```python
from build123d import *

# Parameters (mm, degrees)
ESQUISSE1_W                  = 38
ESQUISSE1_H                  = 36
BOSS_EXTRU_1_DEPTH           = 3
BOSS_EXTRU_2_DEPTH           = 10
ENL_V_MAT_EXTRU_1_DEPTH      = 54.935146241
ENL_V_MAT_EXTRU_1_DEPTH_BACK = 54.935146241
ESQUISSE4_R                  = 0.75
ENL_V_MAT_EXTRU_2_DEPTH      = 19.8
ENL_V_MAT_EXTRU_3_DEPTH      = 54.935146241
ENL_V_MAT_EXTRU_3_DEPTH_BACK = 54.935146241
ESQUISSE5_R                  = 0.75
BOSS_EXTRU_3_START           = -2.6
BOSS_EXTRU_3_DEPTH           = 30.8
BOSS_EXTRU_4_START           = -19.8
BOSS_EXTRU_4_DEPTH           = 19.8


with BuildPart() as part:
    # Esquisse1 → Boss.-Extru.1 (new body)
    with BuildSketch(Plane.XY):
        with Locations((19, 18)):
            Rectangle(ESQUISSE1_W, ESQUISSE1_H)
    extrude(amount=BOSS_EXTRU_1_DEPTH)

    # Esquisse2 → Boss.-Extru.2 (add)
    with BuildSketch(Plane.XY.offset(3)):
        Polygon((38, 33.1), (3, 33.1), (3, 2.9), (38, 2.9), (38, 0), (0, 0), (0, 36), (38, 36), align=None)
    extrude(amount=BOSS_EXTRU_2_DEPTH)

    # Esquisse3 → Enlèv. mat.-Extru.1 (cut, two sides: drawn at the far end of the back side and taken through both)
    with BuildSketch(Plane(origin=(0, 0, 0), x_dir=(-1, 0, 0), z_dir=(0, 0, -1)).offset(-ENL_V_MAT_EXTRU_1_DEPTH_BACK)):
        Polygon((0, 2.6), (0, 0), (-18.2, 0), (-18.2, 5.809151049), align=None)
        Polygon((-18.2, 36), (-18.2, 30.190848951), (0, 33.4), (0, 36), align=None)
    extrude(amount=ENL_V_MAT_EXTRU_1_DEPTH + ENL_V_MAT_EXTRU_1_DEPTH_BACK, mode=Mode.SUBTRACT)

    # Esquisse4 → Enlèv. mat.-Extru.2 (cut)
    with BuildSketch(Plane(origin=(38, 0, 0), x_dir=(0, 0, -1), z_dir=(1, 0, 0))):
        with Locations((-3, 2.9)):
            Circle(ESQUISSE4_R)
        with Locations((-3, 33.1)):
            Circle(ESQUISSE4_R)
    extrude(amount=-ENL_V_MAT_EXTRU_2_DEPTH, mode=Mode.SUBTRACT)

    # Esquisse5 → Enlèv. mat.-Extru.3 (cut, two sides: drawn at the far end of the back side and taken through both)
    with BuildSketch(Plane.XZ.offset(-ENL_V_MAT_EXTRU_3_DEPTH_BACK)):
        with Locations((3, 3)):
            Circle(ESQUISSE5_R)
    extrude(amount=ENL_V_MAT_EXTRU_3_DEPTH + ENL_V_MAT_EXTRU_3_DEPTH_BACK, mode=Mode.SUBTRACT)

    # Esquisse6 → Boss.-Extru.3 (add)
    with BuildSketch(Plane.XZ.offset(BOSS_EXTRU_3_START)):
        Polygon((0, 0), (0, 13), (-2, 0), align=None)
    extrude(amount=-BOSS_EXTRU_3_DEPTH)

    # Esquisse7 → Boss.-Extru.4 (add)
    with BuildSketch(Plane(origin=(38, 0, 0), x_dir=(0, 0, -1), z_dir=(1, 0, 0)).offset(BOSS_EXTRU_4_START)):
        Polygon((0, 0), (-13, 0), (0, -2), align=None)
        Polygon((0, 38), (0, 36), (-13, 36), align=None)
    extrude(amount=BOSS_EXTRU_4_DEPTH)


solid = part.part
```
Model file for the job. Use its own axes, mm. A direction names the side the tool comes from. Give positions to 0.01 mm unless a question says otherwise; leave off trailing zeros. Loops run counter-clockwise (first coordinate to the right, second up) from the corner with the lowest first, then second, coordinate; pieces in that order, holes last. Notation, with made-up numbers: (3, -12) -> (39, -12) arc R34 ccw to (39, 27) -> close; hole circle Ø6 at (3, 43.25). An arc over 180 degrees is marked (long way). Use CSV: the item, a comma, the result in double quotes. Start each with the question number.
1) Slice it at D-D on z = 4.5. Give the cut face in (x, y), plus the area to 3 significant figures.
2) Mould opens along Y. For faces 4 (the flat face through (28, 2.9, 8)), 5 (the flat face through (-1, 33.4, 4)), 6 (the flat face through (18.2, 1, 5)) say: released by +Y, released by -Y, zero draft, split by the parting line, or undercut.
3) Tool access for faces 1 (the flat face through (18.2, 35, 5)), 2 (the flat face through (28, 33.1, 8)), 3 (the flat face through (-1, 2.6, 4)): list every direction of +Z, -Z, +X, -X, +Y, -Y with a clear straight run to the whole face (end or side of a thin tool).
4) Slice it at C-C on y = 9.5. Give the cut face in (x, z).
5) Slice it at A-A on x = 24.5. Give the cut face in (y, z), plus the area to 3 significant figures.
6) Wall check: line 1 (Y direction, x = 27.5, z = 8.5); line 2 (X direction, y = 2, z = 5.5); line 3 (Z direction, x = 4, y = 13.5). Give the ranges that are in metal, low to high.
7) Flat gauge pins, fed straight in: pin 1 Ø3 at (x, y) = (30.5, 5.5) entering from +Z; pin 2 Ø7.5 at (x, z) = (25.5, 9) entering from -Y; pin 3 Ø6 at (y, z) = (22, 7.5) entering from -X. Where does each tip first touch, or does it go through?
8) Slice it at B-B on z = 10.25. Give the cut face in (x, y).
Computed values:
1,outline,"(-1.31, 2.6) -> (0, 2.6) -> (3, 3.13) -> (3, 32.87) -> (0, 33.4) -> (-1.31, 33.4) -> close; (18.2, -1.31) -> (38, -1.31) -> (38, 2.9) -> (18.2, 2.9) -> close; (18.2, 33.1) -> (38, 33.1) -> (38, 37.31) -> (18.2, 37.31) -> close"
1,area,"298 mm^2"
2,face 4,"undercut"
2,face 5,"released by +Y"
2,face 6,"zero draft"
3,face 1,"+Z, -Z, +Y"
3,face 2,"+Z, +X"
3,face 3,"+Z, -Z, -X, -Y"
4,outline,"(-2, 0) -> (38, 0) -> (38, 3) -> (3.75, 3) arc R0.75 cw (long way) to (3, 3.75) -> (3, 13) -> (0, 13) -> close"
5,outline,"(-2, 0) -> (38, 0) -> (36, 13) -> (33.1, 13) -> (33.1, 3.75) arc R0.75 cw (long way) to (32.35, 3) -> (3.65, 3) arc R0.75 cw (long way) to (2.9, 3.75) -> (2.9, 13) -> (0, 13) -> close"
5,area,"189 mm^2"
6,line 1,"y = -0.69 to 2.9, 33.1 to 36.69"
6,line 2,"x = 18.2 to 38"
6,line 3,"z = 0 to 3"
7,pin 1,"stops at z = 3"
7,pin 2,"stops at y = -1.19"
7,pin 3,"stops at x = -1.31"
8,outline,"(-0.42, 2.6) -> (0, 2.6) -> (3, 3.13) -> (3, 32.87) -> (0, 33.4) -> (-0.42, 33.4) -> close; (18.2, -0.42) -> (38, -0.42) -> (38, 2.9) -> (18.2, 2.9) -> close; (18.2, 33.1) -> (38, 33.1) -> (38, 36.42) -> (18.2, 36.42) -> close"
